Could you check a few things on this drawing? It's one solid part, dimensions in mm from its lowest x, y, z. Give positions to 0.01 mm unless a question says otherwise; leave off trailing zeros. Order: outer loops, then holes, each group sorted by start corner. A loop starts at its lowest first (then second) coordinate and runs counter-clockwise, first axis right, second up.
(1) Will these pins go through, and if not, where does the flat tip stop? pin 1 (1.6 mm diameter, centred on x = 34.5, z = 6.5, fed in from +Y); pin 2 (3 mm diameter, centred on x = 53.4, y = 5.75, fed in from -Z).
(2) If we mould it in two halves opening along Y, with no side actions, what happens to the marked faces 1, 2, 3 and 4? For each: released by +Y, released by -Y, zero draft, split by the parting line, or undercut.
(3) Imagine slicing it at D-D, the plane y = 5.75. Write out the boundary of the cut face in (x, z).
(4) Imagine slicing it at A-A, the plane y = 2. Write out the boundary of the cut face in (x, z), then the cut area to 3 significant figures.
(5) Imagine slicing it at B-B, the plane x = 6. Write out the boundary of the cut face in (y, z).
(6) If I drill on probe 1 along X at (y, z) = (1.6, 2.5); probe 2 along Y at (x, z) = (2.6, 6.2); probe 3 along X at (y, z) = (30, 6), over which ranges is the centre line in solid material (lowest first)?
(7) Imagine slicing it at C-C, the plane z = 2.5. Write out the boundary of the cut face in (x, y).
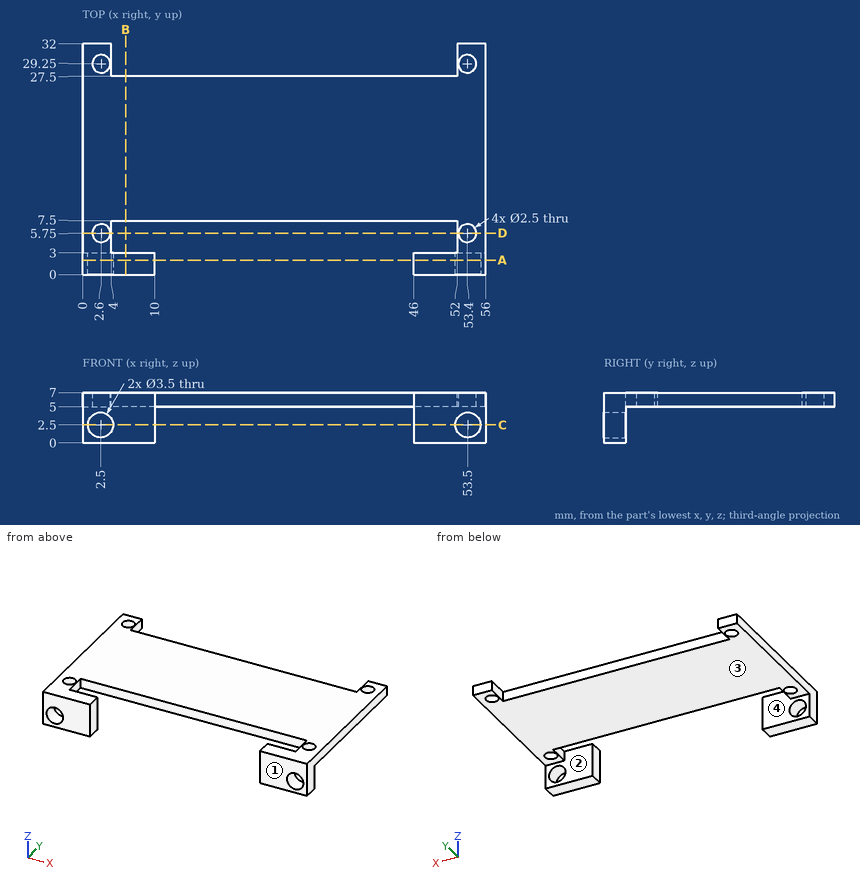
Answer block:
1. pin 1: stops at y = 27.5
1. pin 2: stops at z = 5
2. face 1: released by -Y
2. face 2: undercut
2. face 3: zero draft
2. face 4: undercut
3. outline: (0, 5) - (1.35, 5) - (1.35, 7) - (0, 7) - close; (3.85, 5) - (4, 5) - (4, 7) - (3.85, 7) - close; (52, 5) - (52.15, 5) - (52.15, 7) - (52, 7) - close; (54.65, 5) - (56, 5) - (56, 7) - (54.65, 7) - close
4. outline: (0, 0) - (10, 0) - (10, 7) - (0, 7) - close; (46, 0) - (56, 0) - (56, 7) - (46, 7) - close; hole circle Ø3.5 at (2.5, 2.5); hole circle Ø3.5 at (53.5, 2.5)
4. area: 121 mm2
5. outline: (0, 0) - (3, 0) - (3, 7) - (0, 7) - close; (7.5, 5) - (27.5, 5) - (27.5, 7) - (7.5, 7) - close
6. probe 1: x = 0 to 0.75, 4.25 to 10, 46 to 51.75, 55.25 to 56
6. probe 2: y = 0 to 4.5, 7 to 28, 30.5 to 32
6. probe 3: x = 0 to 1.6, 3.6 to 4, 52 to 52.4, 54.4 to 56
7. outline: (0, 0) - (0.75, 0) - (0.75, 3) - (0, 3) - close; (4.25, 0) - (10, 0) - (10, 3) - (4.25, 3) - close; (46, 0) - (51.75, 0) - (51.75, 3) - (46, 3) - close; (55.25, 0) - (56, 0) - (56, 3) - (55.25, 3) - close
